Work out the finished part from the listing and answer in its coordinate system (mm). A direction names the side the tool comes from. Coordinates: 2 decimals unless noted, no trailing zeros. Write each loop counter-clockwise with the first axis right and the second up, starting at its lowest first coordinate (ties: lowest second). Pieces come first, ordered by that corner, then holes. Notation, with made-up numbers: (58.25, -1.75) - (83.25, -1.75) arc R12 ccw to (83.25, 14.25) - close; hole circle Ø9 at (4.25, 52.25). An arc over 180 degrees is marked (long way). Use a Markdown table: item, result. Add a question column.
(1) Given pin 1 Ø3 at (x, y) = (-14, 18) entering from +Z; pin 2 Ø10 at (y, z) = (32, 5) entering from -X; pin 3 Ø3 at (x, z) = (-7.5, 6) entering from +Y; pin 4 Ø6 at (y, z) = (13, -12.5) entering from -X, each flat-ended and moving along its own axis, determine where each tip first touches the part or whether it passes through.
(2) A tool of negligible diameter and unlimited length cuts with its end or side. For faces 4 (the face through (8.03, 30, 7.88)), 5 (the face through (-22.713, 24.185, -6.086)), 6 (the face through (-22.69, 24.18, 6.08)), from which of +Z, -Z, +X, -X, +Y, -Y can it reach the whole face along a straight path? Write none if from no direction.
(3) Find the intervals of material crossed by line 1 (X direction, y = 35, z = -4.5); line 2 (X direction, y = 9.5, z = 5); line 3 (Z direction, x = 2, y = 23), in increasing order. Write a range as from..to.
(4) The part is cut by section A-A, the plane y = 9. Give the vertices of the cut face in (x, z), then the cut area to 3 significant figures.
(5) For a pull along Z with two mould halves and no side action, classify faces 1 (the face through (21.44, 0, -7.44)), 2 (the face through (-24.5, 24.8, 0.1)), 3 (the face through (1.54, 32.21, -17.58)) as released by +Z, released by -Z, zero draft, split by the parting line, or undercut.
(6) The part is cut by section B-B, the plane x = 3.5. Give the vertices of the cut face in (y, z), then the cut area to 3 significant figures.
(7) The part is cut by section C-C, the plane z = 4. Give the vertices of the cut face in (x, y) (3 decimals).
from build123d import *

# Parameters (mm, degrees)
ESBO_O1_R                = 31.5
ESBO_O1_R_2              = 22.5
RESSALTO_EXTRUS_O1_DEPTH = 2
RESSALTO_EXTRUS_O2_DEPTH = 45
REVOLU_O1_ANGLE          = 10
PADR_OCIRCULAR1_COUNT    = 2
PADR_OCIRCULAR1_ANGLE    = 90
ESBO_O5_R                = 11.25
ESBO_O5_R_2              = 10.25
RESSALTO_EXTRUS_O3_DEPTH = 26.37477


with BuildPart() as part:
    # Esboço1 → Ressalto-extrusão1 (new body)
    with BuildSketch(Plane(origin=(0, 0, 0), x_dir=(1, 0, 0), z_dir=(0, 1, 0))):
        with Locations(Location((0, 0, 0), (0, 0, 270))):
            Circle(ESBO_O1_R)
        with Locations(Location((0, 0, 0), (0, 0, 270))):
            Circle(ESBO_O1_R_2, mode=Mode.SUBTRACT)
    extrude(amount=RESSALTO_EXTRUS_O1_DEPTH)

    # Esboço3 → Ressalto-extrusão2 (add)
    with BuildSketch(Plane(origin=(0, 2, 0), x_dir=(1, 0, 0), z_dir=(0, 1, 0))):
        with BuildLine():
            Line((-5.823428515, -21.733331092), (-6.341066605, -23.665182744))
            ThreePointArc((-6.341066605, -23.665182744), (0, -24.5), (6.341066605, -23.665182744))
            Line((6.341066605, -23.665182744), (5.823428515, -21.733331092))
            ThreePointArc((5.823428515, -21.733331092), (0, -22.5), (-5.823428515, -21.733331092))
        make_face()
        with BuildLine():
            Line((-21.733331092, -5.823428515), (-23.665182744, -6.341066605))
            ThreePointArc((-23.665182744, -6.341066605), (-24.5, 0), (-23.665182744, 6.341066605))
            Line((-23.665182744, 6.341066605), (-21.733331092, 5.823428515))
            ThreePointArc((-21.733331092, 5.823428515), (-22.5, 0), (-21.733331092, -5.823428515))
        make_face()
        with BuildLine():
            Line((-5.823428515, 21.733331092), (-6.341066605, 23.665182744))
            ThreePointArc((-6.341066605, 23.665182744), (0, 24.5), (6.341066605, 23.665182744))
            Line((6.341066605, 23.665182744), (5.823428515, 21.733331092))
            ThreePointArc((5.823428515, 21.733331092), (0, 22.5), (-5.823428515, 21.733331092))
        make_face()
        with BuildLine():
            Line((21.733331092, 5.823428515), (23.665182744, 6.341066605))
            ThreePointArc((23.665182744, 6.341066605), (24.5, 0), (23.665182744, -6.341066605))
            Line((23.665182744, -6.341066605), (21.733331092, -5.823428515))
            ThreePointArc((21.733331092, -5.823428515), (22.5, 0), (21.733331092, 5.823428515))
        make_face()
    extrude(amount=RESSALTO_EXTRUS_O2_DEPTH)

    # Esboço4 → Revolução1 (revolve, symmetric)
    with BuildSketch(Plane.XY) as revolu_o1_sk:
        with BuildLine():
            Line((-24.5, 47), (-21.733331092, 47))
            ThreePointArc((-21.733331092, 47), (-16.270987924, 44.302599501), (-10.25, 43.374770442))
            Line((-10.25, 43.374770442), (-10.25, 17))
            Line((-10.25, 17), (-24.5, 17))
            Line((-24.5, 17), (-24.5, 47))
        make_face()
        with BuildLine():
            Line((10.25, 17), (24.5, 17))
            Line((24.5, 17), (24.5, 47))
            Line((24.5, 47), (21.733331092, 47))
            ThreePointArc((21.733331092, 47), (16.270987924, 44.302599501), (10.25, 43.374770442))
            Line((10.25, 43.374770442), (10.25, 17))
        make_face()
    revolu_o1 = revolve(axis=Axis((0, 0, 0), (0, 1, 0)), revolution_arc=REVOLU_O1_ANGLE / 2)
    revolu_o1 = revolu_o1 + revolve(revolu_o1_sk.sketch, axis=Axis((0, 0, 0), (0, -1, 0)), revolution_arc=REVOLU_O1_ANGLE / 2)

    # PadrãoCircular1: Revolução1 ×2 about axis
    padr_ocircular1_axis = Axis((0, 0, 0), (0, 1, 0))
    for i in range(1, PADR_OCIRCULAR1_COUNT):
        add(revolu_o1.rotate(padr_ocircular1_axis, i * PADR_OCIRCULAR1_ANGLE / (PADR_OCIRCULAR1_COUNT - 1)))

    # Esboço5 → Ressalto-extrusão3 (add)
    with BuildSketch(Plane.XZ.offset(-17)):
        Circle(ESBO_O5_R)
        Circle(ESBO_O5_R_2, mode=Mode.SUBTRACT)
    extrude(amount=-RESSALTO_EXTRUS_O3_DEPTH)


solid = part.part
Model answer:
| question | item | result |
|---|---|---|
| 1 | pin 1 | z = 1.36 |
| 1 | pin 2 | x = -24.5 |
| 1 | pin 3 | y = 43.37 |
| 1 | pin 4 | through |
| 2 | face 4 | +Y, -Y |
| 2 | face 5 | -Z, +Y |
| 2 | face 6 | +Z, +Y |
| 3 | line 1 | -24.08..-22.05, -10.31..-9.21, 9.21..10.31, 22.05..24.08 |
| 3 | line 2 | -23.98..-21.94, 21.94..23.98 |
| 3 | line 3 | -24.42..-22.41, -11.07..-10.05, 10.05..11.07, 22.41..24.42 |
| 4 | outline | (-23.67, -6.34) - (-21.73, -5.82) arc R22.5 cw to (-21.73, 5.82) - (-23.67, 6.34) arc R24.5 ccw to start; (-6.34, -23.67) arc R24.5 ccw to (6.34, -23.67) - (5.82, -21.73) arc R22.5 cw to (-5.82, -21.73) - close; (-6.34, 23.67) - (-5.82, 21.73) arc R22.5 cw to (5.82, 21.73) - (6.34, 23.67) arc R24.5 ccw to start; (21.73, -5.82) - (23.67, -6.34) arc R24.5 ccw to (23.67, 6.34) - (21.73, 5.82) arc R22.5 cw to start |
| 4 | area | 98.4 mm^2 |
| 5 | face 1 | zero draft |
| 5 | face 2 | split by the parting line |
| 5 | face 3 | undercut |
| 6 | outline | (0, -31.3) - (2, -31.3) - (2, -24.25) - (47, -24.25) - (47, -22.23) - (0, -22.23) - close; (0, 22.23) - (47, 22.23) - (47, 24.25) - (2, 24.25) - (2, 31.3) - (0, 31.3) - close; (17, -10.69) - (43.37, -10.69) - (43.37, -9.63) - (17, -9.63) - close; (17, 9.63) - (43.37, 9.63) - (43.37, 10.69) - (17, 10.69) - close |
| 6 | area | 274 mm^2 |
| 7 | outline | (-31.245, 0) - (-22.142, 0) - (-22.142, 47) - (-24.171, 47) - (-24.171, 2) - (-31.245, 2) - close; (-10.515, 17) - (-9.437, 17) - (-9.437, 43.375) - (-10.515, 43.375) - close; (9.437, 17) - (10.515, 17) - (10.515, 43.375) - (9.437, 43.375) - close; (22.142, 0) - (31.245, 0) - (31.245, 2) - (24.171, 2) - (24.171, 47) - (22.142, 47) - close |
